```python
from build123d import *

# Parameters (mm, degrees)
F1_DEPTH = 25


with BuildPart() as f1:
    # F0 (on Front) → F1 (new body)
    with BuildSketch(Plane.XZ):
        with BuildLine():
            ThreePointArc((9.682458, 7.5), (6.123724, 2.094306), (0, 0))
            Line((0, 0), (15, 0))
            Line((15, 0), (20, 5))
            Line((20, 5), (20, 7.5))
            Line((20, 7.5), (9.682458, 7.5))
        make_face()
        with BuildLine():
            ThreePointArc((-9.682458, 7.5), (-6.123724, 2.094306), (0, 0))
            ThreePointArc((0, 0), (6.123724, 2.094306), (9.682458, 7.5))
            Line((9.682458, 7.5), (4.330127, 7.5))
            ThreePointArc((4.330127, 7.5), (0, 5), (-4.330127, 7.5))
            Line((-4.330127, 7.5), (-9.682458, 7.5))
        make_face()
        with BuildLine():
            ThreePointArc((-9.682458, 12.5), (-10, 10), (-9.682458, 7.5))
            Line((-9.682458, 7.5), (-4.330127, 7.5))
            ThreePointArc((-4.330127, 7.5), (-5, 10), (-4.330127, 12.5))
            Line((-4.330127, 12.5), (-9.682458, 12.5))
        make_face()
        with BuildLine():
            Line((4.330127, 7.5), (9.682458, 7.5))
            Line((9.682458, 7.5), (20, 7.5))
            Line((20, 7.5), (20, 12.5))
            Line((20, 12.5), (9.682458, 12.5))
            Line((9.682458, 12.5), (4.330127, 12.5))
            ThreePointArc((4.330127, 12.5), (4.829629, 11.294095), (5, 10))
            ThreePointArc((5, 10), (4.829629, 8.705905), (4.330127, 7.5))
        make_face()
        with BuildLine():
            ThreePointArc((0, 20), (-6.123724, 17.905694), (-9.682458, 12.5))
            Line((-9.682458, 12.5), (-4.330127, 12.5))
            ThreePointArc((-4.330127, 12.5), (0, 15), (4.330127, 12.5))
            Line((4.330127, 12.5), (9.682458, 12.5))
            ThreePointArc((9.682458, 12.5), (6.123724, 17.905694), (0, 20))
        make_face()
        with BuildLine():
            Line((15, 20), (0, 20))
            ThreePointArc((0, 20), (6.123724, 17.905694), (9.682458, 12.5))
            Line((9.682458, 12.5), (20, 12.5))
            Line((20, 12.5), (20, 15))
            Line((20, 15), (15, 20))
        make_face()
    extrude(amount=F1_DEPTH)


solid = f1.part
```
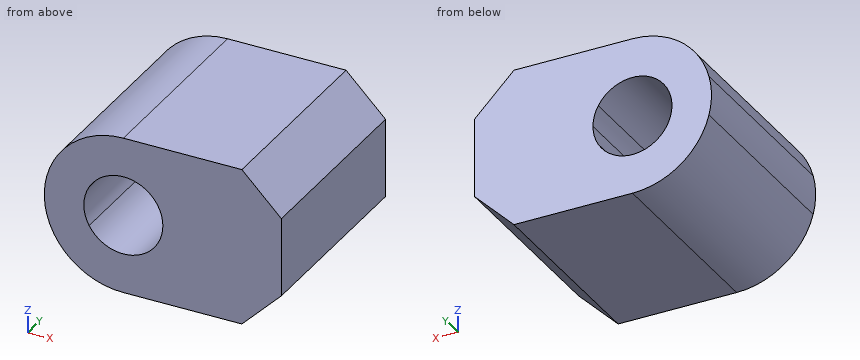
Geometry check sheet. Reference: the model listing, model coordinates, mm. Coordinates: 2 decimals unless noted, no trailing zeros. Write each loop counter-clockwise with the first axis right and the second up, starting at its lowest first coordinate (ties: lowest second). Pieces come first, ordered by that corner, then holes. Notation, with made-up numbers: M -2,51 L 35,51 A25 cw 35,78 Z; hole C -32,23.25 d3. An arc over 180 degrees is marked long. One line per item, written item: value. Start each with the question number.
(1) Depth check by flat-ended pin: pin 1 (1.5 mm diameter, centred on y = -19.5, z = 11.5, fed in from -X). Enter the tip coordinate at first touch or a pass-through.
(2) Sectioned sample at B-B, the plane y = -22.5. Enter the section's corners in (x, z), and give its area (3 significant figures).
(3) Scan lines: line 1 along X through (y, z) = (-15.75, 14.25); line 2 along X through (y, z) = (-12.25, 6.25); line 3 along Z through (x, y) = (2.75, -19.5). Record each from-to range of solid material in increasing order. Write a range as [from, to].
(4) Sectioned sample at C-C, the plane z = 6.25. Enter the section's corners in (x, y), and give its area (3 significant figures).
(5) Sectioned sample at D-D, the plane z = 2. Enter the section's corners in (x, y).
(6) Sectioned sample at A-A, the plane x = 3. Enter the section's corners in (y, z).
Filled sheet:
1. pin 1: x = -9.97
2. outline: M -9.68,7.5 A10 ccw 0,0 L 15,0 L 20,5 L 20,15 L 15,20 L 0,20 A10 ccw -9.68,12.5 A10 ccw Z; hole M 4.33,7.5 A5 ccw 5,10 A5 ccw 4.33,12.5 A5 ccw long Z
2. area: 454 mm²
3. line 1: [-9.05, -2.63], [2.63, 20]
3. line 2: [-9.27, -3.31], [3.31, 20]
3. line 3: [0, 5.82], [14.18, 20]
4. outline: M -9.27,-25 L -3.31,-25 L -3.31,0 L -9.27,0 Z; M 3.31,-25 L 20,-25 L 20,0 L 3.31,0 Z
4. area: 566 mm²
5. outline: M -6,-25 L 17,-25 L 17,0 L -6,0 Z
6. outline: M -25,0 L 0,0 L 0,6 L -25,6 Z; M -25,14 L 0,14 L 0,20 L -25,20 Z
